from build123d import *

# Parameters (mm, degrees)
F1_DEPTH  = 15
F2_W      = 3
F2_H      = 310
F3_DEPTH  = 25
F4_R      = 2.5
F5_DEPTH  = 3
F6_W      = 1
F6_H      = 0.5
F7_DEPTH  = 3
F8_R      = 1
F9_R      = 2.5
F9_R_2    = 1.2
F10_DEPTH = 3
F11_R     = 1.2
F12_DEPTH = 34.2
F13_DEPTH = 3
F14_DEPTH = 3
F15_R     = 2


with BuildPart() as f1:
    # F0 (on Right) → F1 (new body)
    with BuildSketch(Plane.YZ):
        Polygon((-7.5968508422, 3), (-7.5968508422, 0), (22.4031491578, 0), (22.4031491578, 318), (19.4031491578, 318), (19.4031491578, 3), align=None)
    extrude(amount=F1_DEPTH)

    # F2 (on face) → F3 (join)
    with BuildSketch(Plane(origin=(0, 22.4031491578, 0), x_dir=(-1, 0, 0), z_dir=(0, 1, 0))):
        with Locations((1.5, 163)):
            Rectangle(F2_W, F2_H)
        with Locations((-16.5, 163)):
            Rectangle(F2_W, F2_H)
    extrude(amount=-F3_DEPTH)

    # F4 (on face) → F5 (cut)
    with BuildSketch(Plane.XY.offset(3)):
        with Locations((7.5, -2.5968508422)):
            Circle(F4_R)
        with Locations((7.5, 12.4031491578)):
            Circle(F4_R)
    extrude(amount=-F5_DEPTH, mode=Mode.SUBTRACT)

    # F6 (on face) → F7 (cut)
    with BuildSketch(Plane.XZ.offset(-19.4031491578)):
        with Locations((0.5, 7.75)):
            Rectangle(F6_W, F6_H)
        with Locations((14.5, 7.75)):
            Rectangle(F6_W, F6_H)
    extrude(amount=-F7_DEPTH, mode=Mode.SUBTRACT)

    # F8
    f8_edges = [f1.edges().sort_by_distance(p)[0] for p in [
        (7.5, 19.403149, 3),
        (7.5, 22.403149, 0),
        (0, 19.403149, 163),
        (-3, 22.403149, 163),
        (18, 22.403149, 163),
        (15, 19.403149, 163),
    ]]
    fillet(f8_edges, radius=F8_R)

    # F9 (on face) → F10 (cut)
    with BuildSketch(Plane.XZ.offset(-19.4031491578)):
        with Locations((7.5, 312)):
            Circle(F9_R)
        with Locations((7.5, 100)):
            Circle(F9_R_2)
        with Locations((7.5, 200)):
            Circle(F9_R_2)
    extrude(amount=-F10_DEPTH, mode=Mode.SUBTRACT)

    # F11 (on face) → F12 (cut)
    with BuildSketch(Plane(origin=(-3, 0, 0), x_dir=(0, -1, 0), z_dir=(-1, 0, 0))):
        with Locations((-12.4031491578, 300)):
            Circle(F11_R)
        with Locations((-12.4031491578, 100)):
            Circle(F11_R)
        with Locations((-12.4031491578, 200)):
            Circle(F11_R)
    extrude(amount=-F12_DEPTH, mode=Mode.SUBTRACT)

    # F13 (add): a face of the model
    f13_faces = [f1.faces().sort_by_distance(p)[0] for p in [
        (0, 9.1577983799, 1.9953507779),
    ]]
    extrude(f13_faces, amount=F13_DEPTH)

    # F14 (add): a face of the model
    f14_faces = [f1.faces().sort_by_distance(p)[0] for p in [
        (15, 9.1577983799, 1.9953507779),
    ]]
    extrude(f14_faces, amount=F14_DEPTH)

    # F15
    f15_edges = [f1.edges().sort_by_distance(p)[0] for p in [
        (-1.5, -2.596851, 8),
        (16.5, -2.596851, 8),
        (-3, -7.596851, 1.5),
        (18, -7.596851, 1.5),
        (-1.5, -2.596851, 318),
        (16.5, -2.596851, 318),
    ]]
    fillet(f15_edges, radius=F15_R)


solid = f1.part
Verification items for the finished model (mm, model axes). A direction names the side the tool comes from. Round coordinates to 2 decimals unless told otherwise and drop trailing zeros. Loops run counter-clockwise (first coordinate to the right, second up) from the corner with the lowest first, then second, coordinate; pieces in that order, holes last. Notation, with made-up numbers: (3.25, 66.5) - (17.25, 66.5) arc R30 ccw to (17.25, 95.5) - close; hole circle Ø8 at (19.25, 12). An arc over 180 degrees is marked (long way). Answer in a Markdown table with one row per item. Add a question column.
Q1. Release check for a two-part mould opening along Y. For faces 1 (the face through (7, 19.403, 163)), 2 (the face through (18, 8, 2)), 3 (the face through (7, 22.403, 157)), 4 (the face through (8.844, 14.511, 1.521)) record: pulls with the +Y half, pulls with the -Y half, needs draft (parallel to the pull), parting line crosses it, or undercut.
Q2. Material ranges on line 1 (Z direction, x = 7.5, y = 21.65); line 2 (Y direction, x = 7.5, z = 2.05); line 3 (Y direction, x = 17.15, z = 200), recorded low to high.
Q3. Section check A-A on z = 288. Enter the section's corners in (x, y), plus the area to 3 significant figures.
Q4. Tool access check on faces 5 (the face through (15, 8, 161)), 6 (the face through (18, 10, 161)), 7 (the face through (7, 6, 3)). Record the directions out of +Z, -Z, +X, -X, +Y, -Y that give a thin tool (end or side, any length) a straight path to the whole face; none if there is none.
Q5. Gauge pin test, flat ends, axial feed: pin 1 (6.5 mm diameter, centred on x = 9, z = 99.5, fed in from -Y); pin 2 (1.4 mm diameter, centred on y = 12.4, z = 100, fed in from +X); pin 3 (2.5 mm diameter, centred on x = 16, z = 148.5, fed in from -Y). Record the tip position at first contact, or that the pin passes through.
Found:
| question | item | result |
|---|---|---|
| 1 | face 1 | pulls with the -Y half |
| 1 | face 2 | needs draft |
| 1 | face 3 | pulls with the +Y half |
| 1 | face 4 | undercut |
| 2 | line 1 | z = 0.03 to 98.8, 101.2 to 198.8, 201.2 to 309.5, 314.5 to 318 |
| 2 | line 2 | y = -7.6 to -5.1, -0.1 to 9.9, 14.9 to 22.4 |
| 2 | line 3 | y = -2.6 to 11.2, 13.6 to 22.39 |
| 3 | outline | (-3, -2.6) - (0, -2.6) - (0, 18.4) arc R1 cw to (1, 19.4) - (14, 19.4) arc R1 cw to (15, 18.4) - (15, -2.6) - (18, -2.6) - (18, 21.4) arc R1 ccw to (17, 22.4) - (-2, 22.4) arc R1 ccw to (-3, 21.4) - close |
| 3 | area | 195 mm² |
| 4 | face 5 | +Z, -Y |
| 4 | face 6 | +Z, -Z, +X, +Y, -Y |
| 4 | face 7 | +X, -X, -Y |
| 5 | pin 1 | stops at y = 19.4 |
| 5 | pin 2 | passes through |
| 5 | pin 3 | stops at y = -2.6 |
